The drawing under review shows one solid part. Ordinate dimensions are in mm from its lowest x, y, z. Coordinates: 2 decimals unless noted, no trailing zeros. Order: outer loops, then holes, each group sorted by start corner. A loop starts at its lowest first (then second) coordinate and runs counter-clockwise, first axis right, second up. Notation, with made-up numbers: (21.5, 10.5) -> (51.5, 10.5) arc R13 ccw to (51.5, 16.5) -> close; hole circle Ø9 at (-8.5, -9.75). An arc over 180 degrees is marked (long way). Write item = value, one per line.
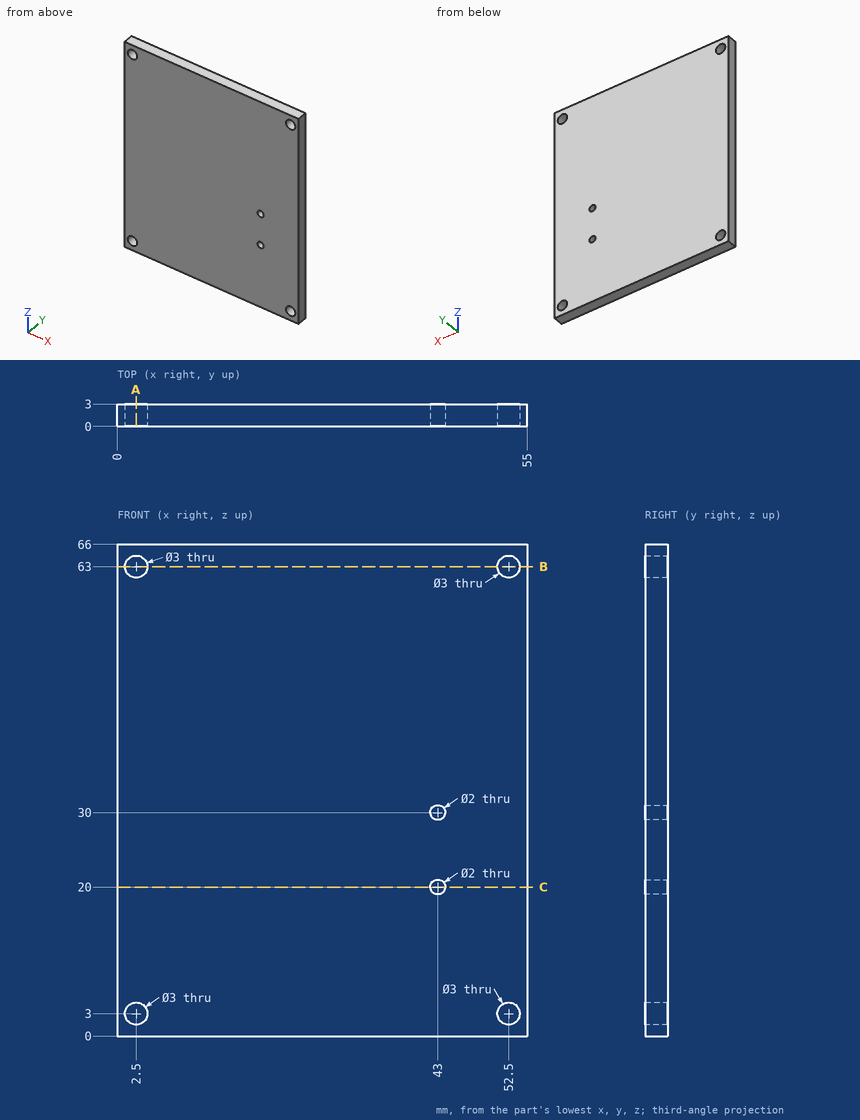
(1) For L1, parallel to X at y = 0.85, z = 3; L2, parallel to X at y = 0.95, z = 62; L3, parallel to X at y = 1.8, z = 30, list the stretches that pass through material, from the lowest coordinate up.
Report:
L1 = 0 to 1, 4 to 51, 54 to 55
L2 = 0 to 1.38, 3.62 to 51.38, 53.62 to 55
L3 = 0 to 42, 44 to 55
(2) We need section A-A (x = 2.5). Write out the cut boundary in (y, z), and give its area (3 significant figures).
Report:
outline = (0, 0) -> (3, 0) -> (3, 1.5) -> (0, 1.5) -> close; (0, 4.5) -> (3, 4.5) -> (3, 61.5) -> (0, 61.5) -> close; (0, 64.5) -> (3, 64.5) -> (3, 66) -> (0, 66) -> close
area = 180 mm²
(3) We need section B-B (z = 63). Write out the cut boundary in (x, y), and give its area (3 significant figures).
Report:
outline = (0, 0) -> (1, 0) -> (1, 3) -> (0, 3) -> close; (4, 0) -> (51, 0) -> (51, 3) -> (4, 3) -> close; (54, 0) -> (55, 0) -> (55, 3) -> (54, 3) -> close
area = 147 mm²
(4) We need section C-C (z = 20). Write out the cut boundary in (x, y).
Report:
outline = (0, 0) -> (42, 0) -> (42, 3) -> (0, 3) -> close; (44, 0) -> (55, 0) -> (55, 3) -> (44, 3) -> close
